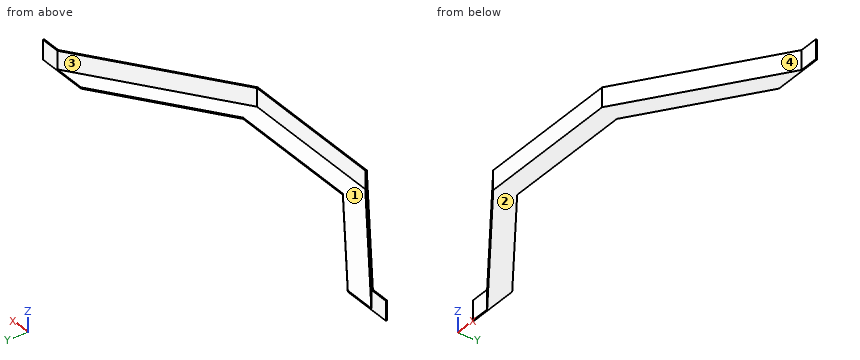
Autodesk Inventor part; units mm, degrees
ref_plane "YZ Plane" through (0, 0, 0) normal (1, 0, 0) x (0, 1, 0)
ref_plane "XZ Plane" through (0, 0, 0) normal (0, 1, 0) x (-1, 0, 0)
ref_plane "XY Plane" through (0, 0, 0) normal (0, 0, 1) x (1, 0, 0)
sketch "Sketch1" plane through (0, 0, 0) normal (0, 0, 1) x (1, 0, 0)
  line L0 (0, 0) -> (190.5, 0)
  line L1 (7.522, 23.8125) -> (182.978, 23.8125)
  line L2 (0, 0) -> (-180.9643, 127)
  line L3 (190.5, 0) -> (371.4643, 127)
  line L4 (-139.5115, 127) -> (7.522, 23.8125)
  line L5 (330.0115, 127) -> (182.978, 23.8125)
  line L6 (-180.9643, 127) -> (-139.5115, 127)
  line L7 (330.0115, 127) -> (371.4643, 127)
  line L8 (-181.4658, 125.4125) -> (-0.5015, -1.5875)
  line L9 (-0.5015, -1.5875) -> (191.0015, -1.5875)
  line L10 (191.0015, -1.5875) -> (371.9658, 125.4125)
  line L11 (-180.9643, 127) -> (-206.3643, 127)
  line L12 (-206.3643, 127) -> (-206.3643, 125.4125)
  line L13 (-206.3643, 125.4125) -> (-181.4658, 125.4125)
  line L14 (371.4643, 127) -> (396.8643, 127)
  line L15 (396.8643, 127) -> (396.8643, 125.4125)
  line L16 (396.8643, 125.4125) -> (371.9658, 125.4125)
  dimension "d0" = 190.5
  dimension "d1" = 23.8125
  dimension "d2" = 23.8125
  dimension "d3" = 23.8125
  dimension "d4" = 144.939
  dimension "d5" = 144.939
  dimension "d6" = 221.0816
  dimension "d7" = 221.0816
  dimension "d8" = 127
  dimension "d9" = 1.5875
  dimension "d10" = 25.4
  dimension "d11" = 1.5875
  dimension "d12" = 25.4
  dimension "d13" = 1.5875
extrude "Extrusion1" add sketch "Sketch1" along normal blind 1.5875 contours L2 L6 L4 L1 L5 L7 L3 L0
extrude "Extrusion2" add sketch "Sketch1" along normal blind 25.4 contours L0 L3 L14 L15 L16 L10 L9 L8 L13 L12 L11 L2
equation "\"d2\" = d1"
equation "\"d3\" = d1"
equation "\"d4\" = d5"
equation "\"d7\" = d6"
properties part number "battery front L"
Model file for the job. Use its own axes, mm. Face numbers are marked on the shaded views. Coordinates: 2 decimals unless noted, no trailing zeros. Write each loop counter-clockwise with the first axis right and the second up, starting at its lowest first coordinate (ties: lowest second). Pieces come first, ordered by that corner, then holes. Notation, with made-up numbers: (36.5, -3) -> (46.5, -3) arc R15 ccw to (46.5, 19) -> close; hole circle Ø3 at (-11, 56). An arc over 180 degrees is marked (long way). One line per item, written item: value. Start each with the question number.
1) Pull direction X, two halves, no side cores. Call the marked faces 1, 2, 3 and 4: +X half, -X half, draft (parallel to the pull), parting line (faces both ways), or undercut.
2) Flat gauge pins, fed straight in: pin 1 Ø7.5 at (x, z) = (380.5, 7.5) entering from -Y; pin 2 Ø12 at (x, z) = (90.5, 9.5) entering from +Y; pin 3 Ø1.5 at (y, z) = (51, 16) entering from +X. Where does each tip first touch, or does it go through?
3) Slice it at D-D on x = -131. Write the cut outline in (y, z), then the cut area to 3 significant figures.
4) Slice it at A-A on z = 6.25. Write the cut outline in (x, y), then the cut area to 3 significant figures.
5) Slice it at C-C on x = 44. Write the cut outline in (y, z), then the cut area to 3 significant figures.
6) Probe probe 1 along Z at (x, y) = (103.5, 12); probe 2 along X at (y, z) = (6.5, 13.75); probe 3 along Y at (x, z) = (131, 21.5). List the from-to ranges inside material, lowest first.
7) Slice it at B-B on y = 107. Write the cut outline in (x, z), then the cut area to 3 significant figures.
Answers follow:
1. face 1: undercut
1. face 2: draft
1. face 3: undercut
1. face 4: +X half
2. pin 1: y = 125.41
2. pin 2: y = 0
2. pin 3: x = 267
3. outline: (90, 0) -> (121.03, 0) -> (121.03, 1.59) -> (91.94, 1.59) -> (91.94, 25.4) -> (90, 25.4) -> close
3. area: 95.4 mm2
4. outline: (-206.36, 125.41) -> (-181.47, 125.41) -> (-0.5, -1.59) -> (191, -1.59) -> (371.97, 125.41) -> (396.86, 125.41) -> (396.86, 127) -> (371.46, 127) -> (190.5, 0) -> (0, 0) -> (-180.96, 127) -> (-206.36, 127) -> close
4. area: 1,090 mm2
5. outline: (-1.59, 0) -> (23.81, 0) -> (23.81, 1.59) -> (0, 1.59) -> (0, 25.4) -> (-1.59, 25.4) -> close
5. area: 78.1 mm2
6. probe 1: 0 to 1.59
6. probe 2: -12.03 to -9.26, 199.76 to 202.53
6. probe 3: -1.59 to 0
7. outline: (-155.23, 0) -> (-111.01, 0) -> (-111.01, 1.59) -> (-152.47, 1.59) -> (-152.47, 25.4) -> (-155.23, 25.4) -> close; (301.51, 0) -> (345.73, 0) -> (345.73, 25.4) -> (342.97, 25.4) -> (342.97, 1.59) -> (301.51, 1.59) -> close
7. area: 272 mm2
